Part model, mm, in its own coordinate system. A direction names the side the tool comes from. Give positions to 0.01 mm unless a question says otherwise; leave off trailing zeros. Order: outer loops, then holes, each group sorted by start corner. A loop starts at its lowest first (then second) coordinate and runs counter-clockwise, first axis right, second up. Notation, with made-up numbers: (-2, -11.5) -> (3, -11.5) arc R21 ccw to (3, 15.5) -> close; hole circle Ø7 at (-28, 61). An arc over 180 degrees is marked (long way). Write item = value, one per line. Start each with the question number.
Item 1: Drill centre lines: line 1 along Y through (x, z) = (-3.25, -2); line 2 along X through (y, z) = (-2.5, 1.25); line 3 along X through (y, z) = (-1.5, 0.25). Where is each one in solid material? Low to high.
Item 2: Tool access for faces 1 (the face through (0, 3, 4)), 2 (the face through (-4.5, 0, 0)), 3 (the face through (-6, 0, 0)), 4 (the face through (-5.55, 0.03, 3.57)): list every direction of +Z, -Z, +X, -X, +Y, -Y with a clear straight run to the whole face (end or side of a thin tool).
Item 3: Band-saw the part on A-A on z = 0. Count the separate pieces of the cut face and the enclosed holes in it, plus the area to 3 significant figures.
Item 4: Flat gauge pins, fed straight in: P1, Ø2.5, axis at x = 9.5, z = 0, coming from the +Y side; P2, Ø1.2, axis at y = -1, z = 0.5, coming from the +X side. Where does each tip first touch, or does it go through?
Item 5: Pull direction Z, two halves, no side cores. Call faces 5 (the face through (8, -3, 0)), 6 (the face through (8, 2, -1)), 7 (the face through (-11, 3, 0)), 8 (the face through (5.55, 0.03, 3.57)): +Z half, -Z half, draft (parallel to the pull), parting line (faces both ways), or undercut.
Item 6: Band-saw the part on B-B on x = 6.5. Write the cut outline in (y, z), plus the area to 3 significant figures.
Item 7: Band-saw the part on C-C on y = 1.75. Write the cut outline in (x, z), plus the area to 3 significant figures.
```python
from build123d import *

# Parameters (mm, degrees)
F0_W     = 24
F0_H     = 8
F1_DEPTH = 4
F2_W     = 6
F2_H     = 4
F3_DEPTH = 25
F4_R     = 1.5
F5_DEPTH = 25
F6_R     = 3
F7_R     = 1.5
F8_W     = 9
F8_H     = 4
F9_DEPTH = 25


with BuildPart() as f1:
    # F0 (on Top) → F1 (new body, symmetric)
    with BuildSketch(Plane.XY):
        Rectangle(F0_W, F0_H)
    extrude(amount=F1_DEPTH, both=True)

    # F2 (on face) → F3 (cut)
    with BuildSketch(Plane.XY.offset(4)):
        with Locations((-9, 0)):
            Rectangle(F2_W, F2_H)
        with Locations((9, 0)):
            Rectangle(F2_W, F2_H)
    extrude(amount=-F3_DEPTH, mode=Mode.SUBTRACT)

    # F4 (on face) → F5 (cut)
    with BuildSketch(Plane.XZ.offset(4)):
        with Locations((-9.5, 0)):
            Circle(F4_R)
        with Locations((9.5, 0)):
            Circle(F4_R)
    extrude(amount=-F5_DEPTH, mode=Mode.SUBTRACT)

    # F6
    f6_edges = [f1.edges().sort_by_distance(p)[0] for p in [
        (12, -3, 4),
        (12, 3, 4),
        (12, -3, -4),
        (12, 3, -4),
        (-12, -3, 4),
        (-12, 3, 4),
        (-12, -3, -4),
        (-12, 3, -4),
    ]]
    fillet(f6_edges, radius=F6_R)

    # F7
    f7_edges = [f1.edges().sort_by_distance(p)[0] for p in [
        (6, 0, 4),
        (-6, 0, 4),
        (6, 0, -4),
        (-6, 0, -4),
    ]]
    fillet(f7_edges, radius=F7_R)

    # F8 (on face) → F9 (cut)
    with BuildSketch(Plane.XY.offset(4)):
        Rectangle(F8_W, F8_H)
    extrude(amount=-F9_DEPTH, mode=Mode.SUBTRACT)


solid = f1.part
```
Values found:
q1.line_1 = -4 to -2, 2 to 4
q1.line_2 = -11.99 to -10.33, -8.67 to 8.67, 10.33 to 11.99
q1.line_3 = -6 to -4.5, 4.5 to 6
q2.face_1 = +Z, +X, -X, +Y, -Y
q2.face_2 = +Z, -Z
q2.face_3 = +Z, -Z, -X
q2.face_4 = +Z, -X
q3.separate_pieces = 5
q3.enclosed_holes = 1
q3.area = 84.0 mm^2
q4.P1 = through
q4.P2 = 6
q5.face_5 = undercut
q5.face_6 = draft
q5.face_7 = undercut
q5.face_8 = +Z half
q6.outline = (-4, -4) -> (-2, -4) -> (-2, 4) -> (-4, 4) -> close; (2, -4) -> (4, -4) -> (4, 4) -> (2, 4) -> close
q6.area = 32.0 mm^2
q7.outline = (-6, -2.5) arc R1.5 ccw to (-4.5, -4) -> (-4.5, 4) arc R1.5 ccw to (-6, 2.5) -> close; (4.5, -4) arc R1.5 ccw to (6, -2.5) -> (6, 2.5) arc R1.5 ccw to (4.5, 4) -> close
q7.area = 22.1 mm^2
